Input: part model. Units: mm. Frame: model coordinates. Face numbers are marked on the shaded views. A direction names the side the tool comes from. Give positions to 0.01 mm unless a question says otherwise; leave off trailing zeros. Write each loop counter-clockwise with the first axis right and the second up, starting at its lowest first coordinate (ties: lowest second). Pieces come first, ordered by that corner, then holes. Notation, with made-up numbers: (6, 17.5) -> (30, 17.5) arc R21 ccw to (30, 53.5) -> close; hole circle Ø5 at (67, 57). An arc over 180 degrees is marked (long way). Return JSON: item names as keys, results as strings. Group by question number.
Item 1: Section A-A, the plane x = 7.5. Return loops of the section in (y, z), then the cut area to 3 significant figures.
Item 2: Set-up query: the marked faces 4 and 5. Return all of +Z, -Z, +X, -X, +Y, -Y with unobstructed straight access to the full face (end or side cutting, diameter ignored); none if empty.
Item 3: Line query: line 1 (Z direction, x = 9, y = 3.5); line 2 (Y direction, x = -5.75, z = 42.5). Output: solid intervals per line, ascending. Write a range as [from, to].
Item 4: Mould query, pull axis Z, two halves, no side actions, for the marked faces 1, 2 and 3. Classes: released by +Z, released by -Z, zero draft, split by the parting line, or undercut.
Item 5: Section B-B, the plane z = 58.5. Return loops of the section in (x, y), then the cut area to 3 significant figures.
Item 6: Pin query (flat end, axial travel): P1, Ø8, axis at x = 4, z = 37.5, coming from the +Y side; P2, Ø1.5, axis at x = 1, z = 63, coming from the -Y side; P3, Ø1.6, axis at y = 0.5, z = 50, coming from the -X side. Return the tip coordinate at first contact, or that it passes through.
from build123d import *

# Parameters (mm, degrees)
F0_R     = 12.5
F1_DEPTH = 2
F2_W     = 2
F2_H     = 11.4599357944
F2_H_2   = 2
F2_W_2   = 11.4599357944
F3_DEPTH = 80
F4_R     = 12.5
F5_DEPTH = 2


with BuildPart() as f1:
    # F0 (on Top) → F1 (new body)
    with BuildSketch(Plane.XY):
        Circle(F0_R)
    extrude(amount=F1_DEPTH)

    # F2 (on face) → F3 (join)
    with BuildSketch(Plane.XY.offset(2)):
        with Locations((0, 6.7299678972)):
            Rectangle(F2_W, F2_H)
        Rectangle(F2_W, F2_H_2)
        with Locations((-6.7299678972, 0)):
            Rectangle(F2_W_2, F2_H_2)
        with Locations((6.7299678972, 0)):
            Rectangle(F2_W_2, F2_H_2)
        with Locations((0, -6.7299678972)):
            Rectangle(F2_W, F2_H)
    extrude(amount=F3_DEPTH)

    # F4 (on face) → F5 (join)
    with BuildSketch(Plane.XY.offset(82)):
        Circle(F4_R)
    extrude(amount=F5_DEPTH)


solid = f1.part
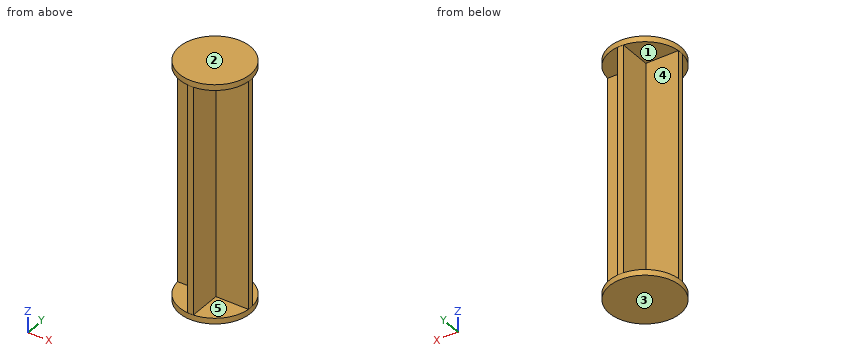
Answer below:
{
 "1": {"outline": "(-10, 0) -> (10, 0) -> (10, 2) -> (1, 2) -> (1, 82) -> (10, 82) -> (10, 84) -> (-10, 84) -> (-10, 82) -> (-1, 82) -> (-1, 2) -> (-10, 2) -> close", "area": "240 mm2"},
 "2": {"face 4": "-X, +Y", "face 5": "+X, -Y"},
 "3": {"line 1": "z = [0, 2], [82, 84]", "line 2": "y = [-1, 1]"},
 "4": {"face 1": "undercut", "face 2": "released by +Z", "face 3": "released by -Z"},
 "5": {"outline": "(-12.46, -1) -> (-1, -1) -> (-1, -12.46) -> (1, -12.46) -> (1, -1) -> (12.46, -1) -> (12.46, 1) -> (1, 1) -> (1, 12.46) -> (-1, 12.46) -> (-1, 1) -> (-12.46, 1) -> close", "area": "95.7 mm2"},
 "6": {"P1": "stops at y = 12.46", "P2": "stops at y = -12.46", "P3": "stops at x = -12.46"}
}
